Input: dimensioned drawing with shaded views. Units: mm. Origin: part minimum x, y, z. Give positions to 0.01 mm unless a question says otherwise; leave off trailing zeros. Write each loop counter-clockwise with the first axis right and the second up, starting at its lowest first coordinate (ties: lowest second). Pieces come first, ordered by that corner, then holes.
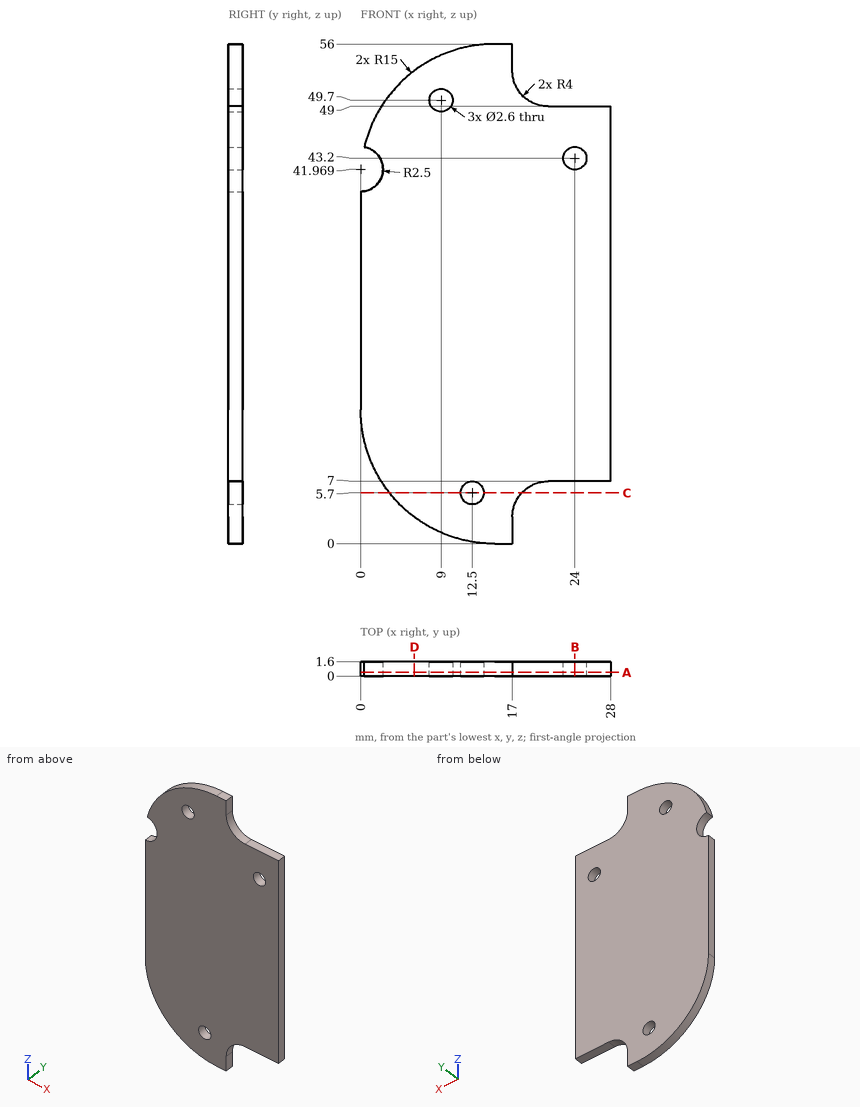
Item 1: Line query: L1, parallel to Z at x = 24, y = 1.1; L2, parallel to Z at x = 9, y = 1; L3, parallel to X at y = 1.25, z = 5.7. Output: solid intervals per line, ascending.
Found:
L1: z = 7 to 41.9, 44.5 to 49
L2: z = 1.25 to 48.4, 51 to 54.75
L3: x = 3.23 to 11.2, 13.8 to 18.05
Item 2: Section C-C, the plane z = 5.7. Return the cut outline in (x, y), plus the area to 3 significant figures.
Found:
outline: (3.23, 0) - (11.2, 0) - (11.2, 1.6) - (3.23, 1.6) - close; (13.8, 0) - (18.05, 0) - (18.05, 1.6) - (13.8, 1.6) - close
area: 19.5 mm2
Item 3: Section D-D, the plane x = 6. Return the cut outline in (y, z), plus the area to 3 significant figures.
Found:
outline: (0, 3) - (1.6, 3) - (1.6, 53) - (0, 53) - close
area: 80.0 mm2
Item 4: Section B-B, the plane x = 24. Return the cut outline in (y, z), plus the area to 3 significant figures.
Found:
outline: (0, 7) - (1.6, 7) - (1.6, 41.9) - (0, 41.9) - close; (0, 44.5) - (1.6, 44.5) - (1.6, 49) - (0, 49) - close
area: 63.0 mm2
Item 5: Pin query (flat end, axial travel): pin 1 Ø0.8 at (x, y) = (25, 1) entering from -Z; pin 2 Ø0.5 at (y, z) = (1, 55) entering from +X. Return the tip coordinate at first contact, or that it passes through.
Found:
pin 1: stops at z = 7
pin 2: stops at x = 17
Item 6: Section A-A, the plane y = 0.4. Return the cut outline in (x, z), plus the area to 3 significant figures.
Found:
outline: (0, 15) arc R15 ccw to (15, 0) - (17, 0) - (17, 3) arc R4 cw to (21, 7) - (28, 7) - (28, 49) - (21, 49) arc R4 cw to (17, 53) - (17, 56) - (15, 56) arc R15 ccw to (0.4, 44.44) arc R2.5 cw to (0, 39.47) - close; hole circle Ø2.6 at (9, 49.7); hole circle Ø2.6 at (12.5, 5.7); hole circle Ø2.6 at (24, 43.2)
area: 1,300 mm2
